from build123d import *

# Parameters (mm, degrees)
BOSS_EXTRUDE1_DEPTH = 139.7
SKETCH2_R           = 2.54
CUT_EXTRUDE1_DEPTH  = 25.4
SKETCH3_R           = 6.35
BOSS_EXTRUDE2_DEPTH = 0.254


with BuildPart() as part:
    # Sketch1 → Boss-Extrude1 (new body)
    with BuildSketch(Plane(origin=(0, 0, 0), x_dir=(1, 0, 0), z_dir=(0, 1, 0))):
        Polygon((7.332348419, 0), (3.666174209, 6.35), (-3.666174209, 6.35), (-7.332348419, 0), (-3.666174209, -6.35), (3.666174209, -6.35), align=None)
    extrude(amount=BOSS_EXTRUDE1_DEPTH)

    # Sketch2 → Cut-Extrude1 (cut)
    with BuildSketch(Plane(origin=(0, 139.7, 0), x_dir=(1, 0, 0), z_dir=(0, 1, 0))):
        Circle(SKETCH2_R)
    extrude(amount=-CUT_EXTRUDE1_DEPTH, mode=Mode.SUBTRACT)

    # Sketch3 → Boss-Extrude2 (add)
    with BuildSketch(Plane.XZ):
        Circle(SKETCH3_R)
    extrude(amount=BOSS_EXTRUDE2_DEPTH)


solid = part.part
For this review, take the finished solid that the model builds, in its own axes (mm). A direction names the side the tool comes from. Coordinates: 2 decimals unless noted, no trailing zeros. Order: outer loops, then holes, each group sorted by start corner. A loop starts at its lowest first (then second) coordinate and runs counter-clockwise, first axis right, second up. Notation, with made-up numbers: (-16.5, 46.5) - (26.5, 46.5) arc R23 ccw to (26.5, 84.5) - close; hole circle Ø5 at (26.5, -21). An arc over 180 degrees is marked (long way). Use one line per item in the form item = value.
Q1. For faces 1 (the cylindrical face through (-0.33, 127.18, -2.52)), 2 (the flat face through (-3, 0, 6)), 3 (the flat face through (-3, 0, -6)), 4 (the flat face through (3, 0, 6)), list the 3-axis set-ups (+Z, -Z, +X, -X, +Y, -Y) from which the entire face can be reached by the end or side of a thin tool; tool diameter is ignored.
Checked values:
face_1 = +Y
face_2 = +Z, -X, -Y
face_3 = -Z, -X, -Y
face_4 = +Z, +X, -Y
Q2. Consider section B-B (z = 1.25). Give the boundary of the cut face in (x, y), then the cut area to 3 significant figures.
Checked values:
outline = (-6.61, 0) - (-6.23, 0) - (-6.23, -0.25) - (6.23, -0.25) - (6.23, 0) - (6.61, 0) - (6.61, 139.7) - (2.21, 139.7) - (2.21, 114.3) - (-2.21, 114.3) - (-2.21, 139.7) - (-6.61, 139.7) - close
area = 1,740 mm2
Q3. For probe 1 along Z at (x, y) = (0, 133.75); probe 2 along X at (y, z) = (131.5, 0); probe 3 along Y at (x, z) = (-1.75, -1.5), list the stretches that pass through material, from the lowest coordinate up. Write a range as from..to.
Checked values:
probe_1 = -6.35..-2.54, 2.54..6.35
probe_2 = -7.33..-2.54, 2.54..7.33
probe_3 = -0.25..114.3
Q4. Consider section A-A (y = 42). Give the boundary of the cut face in (x, z), then the cut area to 3 significant figures.
Checked values:
outline = (-7.33, 0) - (-3.67, -6.35) - (3.67, -6.35) - (7.33, 0) - (3.67, 6.35) - (-3.67, 6.35) - close
area = 140 mm2
Q5. For P1, Ø6, axis at y = 108.5, z = 3.5, coming from the +X side; P2, Ø2, axis at x = 5.5, y = 54.5, coming from the -Z side, all flat-tipped, find the tip position at first contact; note any pin that passes through.
Checked values:
P1 = 7.04
P2 = -4.91
Q6. Draft analysis for pull direction Z (two halves, no side actions). For faces 5 (the flat face through (5.525, 68.872, -3.131)), 6 (the flat face through (3, 0, -6)), 7 (the flat face through (0, 114.3, 0)), 8 (the flat face through (0, 69, 6.35)), state which applies: +Z half, -Z half, draft (parallel to the pull), parting line (faces both ways), or undercut.
Checked values:
face_5 = -Z half
face_6 = draft
face_7 = undercut
face_8 = +Z half
